Can you work these out from the model? Positions are in its coordinate system, mm. Face numbers are marked on the shaded views. A direction names the side the tool comes from. Round coordinates to 2 decimals unless told otherwise and drop trailing zeros. Write each loop counter-clockwise with the first axis right and the second up, starting at its lowest first coordinate (ties: lowest second). Pieces come first, ordered by that corner, then holes. Notation, with made-up numbers: (69.25, -26.75) -> (92.25, -26.75) arc R25 ccw to (92.25, 8.25) -> close; hole circle Ø4 at (18, 58). An arc over 180 degrees is marked (long way). Use CSV: the item, a comma, the result in double quotes.
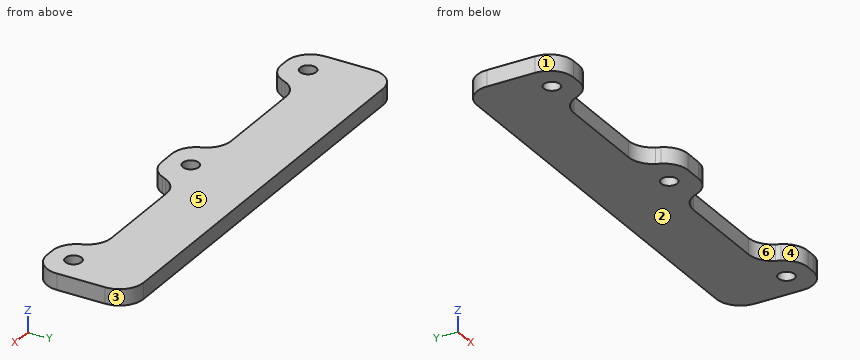
```python
from build123d import *

# Parameters (mm, degrees)
F1_DEPTH = 25.4
F2_R     = 38.1
F4_D     = 25.4


with BuildPart() as f1:
    # F0 (on Top) → F1 (new body)
    with BuildSketch(Plane.XY):
        with BuildLine():
            Line((355.6, 0), (-355.6, 0))
            Line((-355.6, 0), (-355.6, -114.3))
            ThreePointArc((-355.6, -114.3), (-344.4407683632, -141.2407683632), (-317.5, -152.4))
            Line((-317.5, -152.4), (-303.6723769368, -152.4))
            ThreePointArc((-303.6723769368, -152.4), (-283.2012618588, -146.4332140855), (-269.1420502507, -130.4017557723))
            Line((-269.1420502507, -130.4017557723), (-265.9695207151, -123.5982442277))
            ThreePointArc((-265.9695207151, -123.5982442277), (-251.910309107, -107.5667859145), (-231.439194029, -101.6))
            Line((-231.439194029, -101.6), (-86.060805971, -101.6))
            ThreePointArc((-86.060805971, -101.6), (-65.589690893, -107.5667859145), (-51.5304792849, -123.5982442277))
            Line((-51.5304792849, -123.5982442277), (-48.3579497493, -130.4017557723))
            ThreePointArc((-48.3579497493, -130.4017557723), (-34.2987381412, -146.4332140855), (-13.8276230632, -152.4))
            Line((-13.8276230632, -152.4), (13.8276230632, -152.4))
            ThreePointArc((13.8276230632, -152.4), (34.2987381412, -146.4332140855), (48.3579497493, -130.4017557723))
            Line((48.3579497493, -130.4017557723), (51.5304792849, -123.5982442277))
            ThreePointArc((51.5304792849, -123.5982442277), (65.589690893, -107.5667859145), (86.060805971, -101.6))
            Line((86.060805971, -101.6), (231.439194029, -101.6))
            ThreePointArc((231.439194029, -101.6), (251.910309107, -107.5667859145), (265.9695207151, -123.5982442277))
            Line((265.9695207151, -123.5982442277), (269.1420502507, -130.4017557723))
            ThreePointArc((269.1420502507, -130.4017557723), (283.2012618588, -146.4332140855), (303.6723769368, -152.4))
            Line((303.6723769368, -152.4), (317.5, -152.4))
            ThreePointArc((317.5, -152.4), (344.4407683632, -141.2407683632), (355.6, -114.3))
            Line((355.6, -114.3), (355.6, 0))
        make_face()
    extrude(amount=F1_DEPTH)

    # F2
    f2_edges = [f1.edges().sort_by_distance(p)[0] for p in [
        (355.6, 0, 12.7),
        (-355.6, 0, 12.7),
    ]]
    fillet(f2_edges, radius=F2_R)

    # F4 (through all)
    with Locations(Plane.XY.offset(25.4)):
        with Locations((-311.15, -114.3), (0, -114.3), (311.15, -114.3)):
            Hole(F4_D / 2)


solid = f1.part
```
Q1. Please list where these lines run through material, in increasing order: probe 1 along X at (y, z) = (-112, 19); probe 2 along Y at (x, z) = (311.15, 20); probe 3 along X at (y, z) = (-36, 9.5).
Resolved:
probe 1,"x = -355.6 to -323.64, -298.66 to -257.6, -59.9 to -12.49, 12.49 to 59.9, 257.6 to 298.66, 323.64 to 355.6"
probe 2,"y = -152.4 to -127, -101.6 to 0"
probe 3,"x = -355.54 to 355.54"
Q2. If we mould it in two halves opening along X, with no side actions, what happens to the marked faces 1, 2, 3 and 4? For each: released by +X, released by -X, zero draft, split by the parting line, or undercut.
Resolved:
face 1,"released by -X"
face 2,"zero draft"
face 3,"released by +X"
face 4,"undercut"
Q3. On a 3-axis mill with a long thin cutter (end or side, diameter ignored), from which of +Z, -Z, +X, -X, +Y, -Y can I reach the whole of each face in a straight line? I mean the marked faces 5 and 6. Say none if no direction works.
Resolved:
face 5,"+Z, +X, -X, +Y, -Y"
face 6,"+Z, -Z, -Y"
Q4. Suppose I cut it at B-B (z = 17). Write out the boundary of the cut face in (x, y), and give its area (3 significant figures).
Resolved:
outline,"(-355.6, -114.3) arc R38.1 ccw to (-317.5, -152.4) -> (-303.67, -152.4) arc R38.1 ccw to (-269.14, -130.4) -> (-265.97, -123.6) arc R38.1 cw to (-231.44, -101.6) -> (-86.06, -101.6) arc R38.1 cw to (-51.53, -123.6) -> (-48.36, -130.4) arc R38.1 ccw to (-13.83, -152.4) -> (13.83, -152.4) arc R38.1 ccw to (48.36, -130.4) -> (51.53, -123.6) arc R38.1 cw to (86.06, -101.6) -> (231.44, -101.6) arc R38.1 cw to (265.97, -123.6) -> (269.14, -130.4) arc R38.1 ccw to (303.67, -152.4) -> (317.5, -152.4) arc R38.1 ccw to (355.6, -114.3) -> (355.6, -38.1) arc R38.1 ccw to (317.5, 0) -> (-317.5, 0) arc R38.1 ccw to (-355.6, -38.1) -> close; hole circle Ø25.4 at (-311.15, -114.3); hole circle Ø25.4 at (0, -114.3); hole circle Ø25.4 at (311.15, -114.3)"
area,"83,500 mm^2"
Q5. Suppose I cut it at A-A (x = -311.15). Write out the boundary of the cut face in (y, z).
Resolved:
outline,"(-152.4, 0) -> (-127, 0) -> (-127, 25.4) -> (-152.4, 25.4) -> close; (-101.6, 0) -> (0, 0) -> (0, 25.4) -> (-101.6, 25.4) -> close"
Q6. Will these pins go through, and if not, where does the flat tip stop? P1, Ø2, axis at y = -27.5, z = 20, coming from the +X side; P2, Ø12.5, axis at x = -176.5, z = 16.5, coming from the -Y side.
Resolved:
P1,"stops at x = 354.37"
P2,"stops at y = -101.6"
Q7. Suppose I cut it at C-C (x = -33.5). Write out the boundary of the cut face in (y, z), and give its area (3 significant figures).
Resolved:
outline,"(-146.93, 0) -> (0, 0) -> (0, 25.4) -> (-146.93, 25.4) -> close"
area,"3,730 mm^2"
